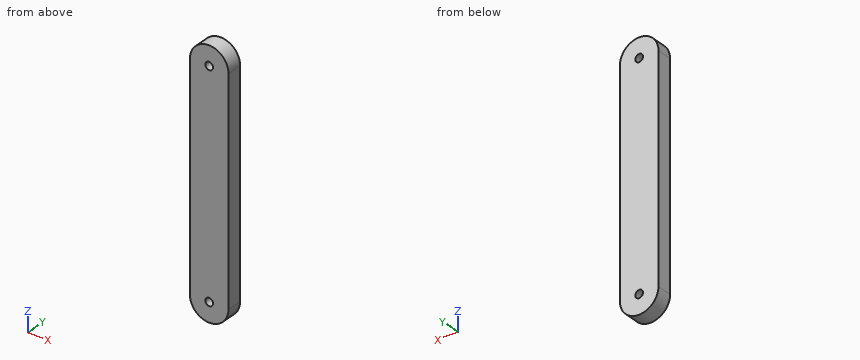
Autodesk Inventor part; units mm, degrees
ref_plane "YZ Plane" through (0, 0, 0) normal (1, 0, 0) x (0, 1, 0)
ref_plane "XZ Plane" through (0, 0, 0) normal (0, 1, 0) x (-1, 0, 0)
ref_plane "XY Plane" through (0, 0, 0) normal (0, 0, 1) x (1, 0, 0)
sketch "Block1" plane through (0, 0, 0) normal (0, 0, 1) x (1, 0, 0)
  line L0 (-25.22, -285) -> (-25.22, 0)
  arc A0 (25.22, 0) -> (-25.22, 0) centre (0, 0) ccw
  line L1 (25.22, 0) -> (25.22, -285)
  arc A1 (-25.22, -285) -> (25.22, -285) centre (0, -285) ccw
  circle A2 centre (0, -285) radius 5.22
  circle A3 centre (0, 0) radius 5.22
  point P0 (0, -142.5)
sketch "Sketch1" plane through (0, 0, 0) normal (0, 1, 0) x (-1, 0, 0)
  arc A0 (-25, 0) -> (25, 0) centre (0, 0) ccw
  arc A1 (25, 285) -> (-25, 285) centre (0, 285) ccw
  line L0 (25, 285) -> (25, 0)
  line L1 (-25, 0) -> (-25, 285)
  circle A2 centre (0, 285) radius 5
  circle A3 centre (0, 0) radius 5
  dimension "d0" = 50
  dimension "d1" = 50
  dimension "d2" = 10
  dimension "d3" = 10
  dimension "d6" = 285
extrude "Extrusion1" add sketch "Sketch1" along normal blind 20
sketch "Sketch2" plane through (0, 20, 0) normal (0, 1, 0) x (1, 0, 0)
  line L0 (25, -285) -> (25, 0)
  line L1 (-25, 0) -> (-25, -285)
  arc A0 (-25, -285) -> (25, -285) centre (0, -285) ccw
  arc A1 (25, 0) -> (-25, 0) centre (0, 0) ccw
  circle A2 centre (0, 0) radius 5
  circle A3 centre (0, -285) radius 5
sketch "DXF" plane through (0, 0, 0) normal (0, 1, 0) x (-1, 0, 0)
  point P0 (0, 0)
equation "\"d6\" = 0.95 * pD"
properties part number "drivelever"
Geometry check sheet. Reference: the model listing, model coordinates, mm. Round coordinates to 2 decimals unless told otherwise and drop trailing zeros. Write each loop counter-clockwise with the first axis right and the second up, starting at its lowest first coordinate (ties: lowest second). Pieces come first, ordered by that corner, then holes.
Item 1: Material ranges on line 1 along Z through (x, y) = (0, 7); line 2 along X through (y, z) = (8.75, 285); line 3 along Z through (x, y) = (4.5, 4), recorded low to high.
Determined:
line 1: z = -25 to -5, 5 to 280, 290 to 310
line 2: x = -25 to -5, 5 to 25
line 3: z = -24.59 to -2.18, 2.18 to 282.82, 287.18 to 309.59
Item 2: Section check C-C (x = 16). Record the boundary of the cut face in (y, z), plus the area to 3 significant figures.
Determined:
outline: (0, -19.21) - (20, -19.21) - (20, 304.21) - (0, 304.21) - close
area: 6,470 mm2
Item 3: Section check D-D (x = -15.5). Record the boundary of the cut face in (y, z).
Determined:
outline: (0, -19.62) - (20, -19.62) - (20, 304.62) - (0, 304.62) - close
Item 4: Section check B-B (y = 4.75). Record the boundary of the cut face in (x, z).
Determined:
outline: (-25, 0) arc R25 ccw to (25, 0) - (25, 285) arc R25 ccw to (-25, 285) - close; hole circle Ø10 at (0, 0); hole circle Ø10 at (0, 285)
Item 5: Go/stop test with flat-tipped pins: pin 1 Ø1 at (x, y) = (1.5, 7.5) entering from -Z; pin 2 Ø3 at (x, y) = (-5, 5) entering from +Z; pin 3 Ø9 at (x, z) = (0, 0) entering from +Y; pin 4 Ø2 at (x, y) = (-3.5, 13) entering from -Z. Record where each tip stops, or that it passes through.
Determined:
pin 1: stops at z = -24.98
pin 2: stops at z = 309.75
pin 3: passes through
pin 4: stops at z = -24.87
Item 6: Section check A-A (x = 0). Record the boundary of the cut face in (y, z), plus the area to 3 significant figures.
Determined:
outline: (0, -25) - (20, -25) - (20, -5) - (0, -5) - close; (0, 5) - (20, 5) - (20, 280) - (0, 280) - close; (0, 290) - (20, 290) - (20, 310) - (0, 310) - close
area: 6,300 mm2
